Could you check a few things on this drawing? It's one solid part, dimensions in mm from its lowest x, y, z. Round coordinates to 2 decimals unless told otherwise and drop trailing zeros. Write each loop counter-clockwise with the first axis right and the second up, starting at its lowest first coordinate (ties: lowest second). Pieces come first, ordered by that corner, then holes. Notation, with made-up numbers: (-12.75, 2.25) - (5.25, 2.25) arc R12 ccw to (5.25, 18.25) - close; hole circle Ø10 at (73, 10). An arc over 180 degrees is marked (long way). Use one line per item in the form item = value. Start each with the question number.
1. Will these pins go through, and if not, where does the flat tip stop? pin 1 (2 mm diameter, centred on x = 5.05, z = 5.05, fed in from -Y); pin 2 (4 mm diameter, centred on x = 14.95, z = 5.05, fed in from +Y).
2. We'd pull the mould along X, two halves only. Please class the marked faces 1, 2 and 3: +X half, -X half, draft (parallel to the pull), parting line (faces both ways), or undercut.
3. I want a section at A-A, the plane x = 10. List the corners of the cut face in (y, z) for me.
4. I want a section at B-B, the plane z = 10. List the corners of the cut face in (x, y) for me.
5. If I drill on line 1 along X through (y, z) = (1.2, 10); line 2 along X through (y, z) = (1.95, 14) (1 decimal); line 3 along X through (y, z) = (0.6, 11), over which ranges is the centre line in solid material (lowest first)?
6. I want a section at C-C, the plane y = 0.35. List the corners of the cut face in (x, z) for me, plus the area to 3 significant figures.
7. I want a section at D-D, the plane x = 15.5. List the corners of the cut face in (y, z) for me.
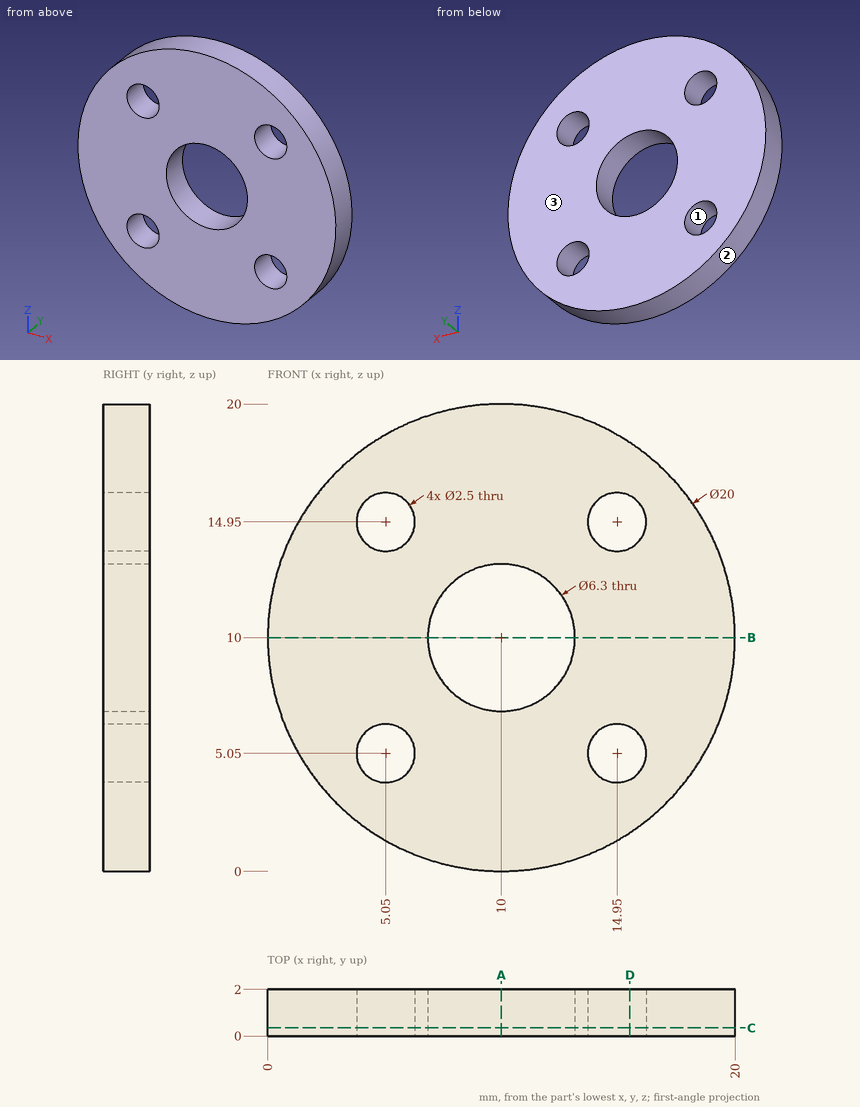
Model answer:
q1.pin_1 = through
q1.pin_2 = 2
q2.face_1 = undercut
q2.face_2 = parting line
q2.face_3 = draft
q3.outline = (0, 0) - (2, 0) - (2, 6.85) - (0, 6.85) - close; (0, 13.15) - (2, 13.15) - (2, 20) - (0, 20) - close
q4.outline = (0, 0) - (6.85, 0) - (6.85, 2) - (0, 2) - close; (13.15, 0) - (20, 0) - (20, 2) - (13.15, 2) - close
q5.line_1 = 0 to 6.85, 13.15 to 20
q5.line_2 = 0.8 to 4.2, 5.9 to 14.1, 15.8 to 19.2
q5.line_3 = 0.05 to 7.01, 12.99 to 19.95
q6.outline = circle Ø20 at (10, 10); hole circle Ø2.5 at (5.05, 5.05); hole circle Ø2.5 at (5.05, 14.95); hole circle Ø6.3 at (10, 10); hole circle Ø2.5 at (14.95, 5.05); hole circle Ø2.5 at (14.95, 14.95)
q6.area = 263 mm2
q7.outline = (0, 1.65) - (2, 1.65) - (2, 3.93) - (0, 3.93) - close; (0, 6.17) - (2, 6.17) - (2, 13.83) - (0, 13.83) - close; (0, 16.07) - (2, 16.07) - (2, 18.35) - (0, 18.35) - close
